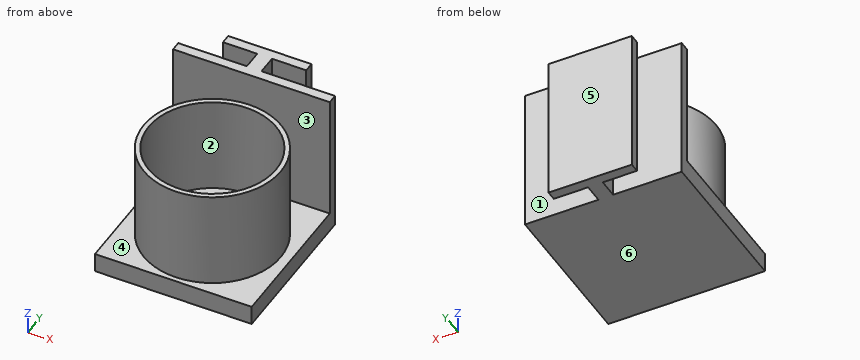
from build123d import *

# Parameters (mm, degrees)
F0_W     = 1.5
F0_H     = 2
F1_DEPTH = 15
F3_DEPTH = 1
F4_W     = 16
F4_H     = 2
F5_DEPTH = 15
F6_R     = 7
F6_R_2   = 6.5
F7_DEPTH = 10


with BuildPart() as f1:
    # F0 (on Top) → F1 (new body)
    with BuildSketch(Plane.XY):
        with Locations((4.5, 7)):
            Rectangle(F0_W, F0_H)
        Polygon((0.25, 8), (3.75, 8), (5.25, 8), (8.75, 8), (8.75, 9), (0.25, 9), align=None)
    extrude(amount=F1_DEPTH)

    # F2 (on face) → F3 (join)
    with BuildSketch(Plane.XZ.offset(-6)):
        Polygon((12.75, 15), (3.75, 15), (-3.25, 15), (-3.25, 0), (12.75, 0), align=None)
    extrude(amount=F3_DEPTH)

    # F4 (on face) → F5 (join)
    with BuildSketch(Plane.XZ.offset(-5)):
        with Locations((4.75, 1)):
            Rectangle(F4_W, F4_H)
    extrude(amount=F5_DEPTH)

    # F6 (on face) → F7 (join)
    with BuildSketch(Plane.XY.offset(2)):
        with Locations((4.75, -2.5)):
            Circle(F6_R)
        with Locations((4.75, -2.5)):
            Circle(F6_R_2, mode=Mode.SUBTRACT)
    extrude(amount=F7_DEPTH)


solid = f1.part
CAD build for the part. Positions are in the model's coordinates, mm. Face numbers are marked on the shaded views. A direction names the side the tool comes from. Round coordinates to 2 decimals unless told otherwise and drop trailing zeros. Write each loop counter-clockwise with the first axis right and the second up, starting at its lowest first coordinate (ties: lowest second). Pieces come first, ordered by that corner, then holes. Notation, with made-up numbers: M -29,54.5 L -9,54.5 A11 cw -9,60.5 Z; hole C 57.25,24 d9. An arc over 180 degrees is marked long. Use a Markdown table: item, result. Add a question column.
1. Slice it at C-C on y = -2.5. Give the cut face in (x, z).
2. Drill centre lines: probe 1 along Y at (x, z) = (4.75, 9.5); probe 2 along Y at (x, z) = (8.5, 14); probe 3 along Y at (x, z) = (2.25, 2.5). Where is each one in solid material? Low to high.
3. Slice it at A-A on z = 4.5. Give the cut face in (x, y), then the cut area to 3 significant figures.
4. Slice it at B-B on x = 8.25. Give the cut face in (y, z).
5. Flat gauge pins, fed straight in: P1, Ø7, axis at x = 1.5, y = -0.5, coming from the +Z side; P2, Ø1, axis at x = 2.5, z = 8.5, coming from the -Y side; P3, Ø4, axis at y = 1.5, z = 9.5, coming from the -X side. Where does each tip first touch, or does it go through?
6. 3-axis set-ups, long thin cutter, end or side, ignore diameter. For the marked faces 1, 2 and 3: which of +Z, -Z, +X, -X, +Y, -Y reach the whole face in a straight line?
7. Pull direction Y, two halves, no side cores. Call the marked faces 4, 5 and 6: released by +Y, released by -Y, zero draft, split by the parting line, or undercut.
8. Slice it at D-D on z = 13.25. Give the cut face in (x, y).
Reply:
| question | item | result |
|---|---|---|
| 1 | outline | M -3.25,0 L 12.75,0 L 12.75,2 L 11.75,2 L 11.75,12 L 11.25,12 L 11.25,2 L -1.75,2 L -1.75,12 L -2.25,12 L -2.25,2 L -3.25,2 Z |
| 2 | probe 1 | y = -9.5 to -9, 4 to 4.5, 5 to 9 |
| 2 | probe 2 | y = 5 to 6, 8 to 9 |
| 2 | probe 3 | y = -9.04 to -8.5, 3.5 to 4.04, 5 to 6, 8 to 9 |
| 3 | outline | M -3.25,5 L 12.75,5 L 12.75,6 L 5.25,6 L 5.25,8 L 8.75,8 L 8.75,9 L 0.25,9 L 0.25,8 L 3.75,8 L 3.75,6 L -3.25,6 Z; C 4.75,-2.5 d14; hole C 4.75,-2.5 d13 |
| 3 | area | 48.7 mm^2 |
| 4 | outline | M -10,0 L 6,0 L 6,15 L 5,15 L 5,2 L 3.56,2 L 3.56,12 L 2.98,12 L 2.98,2 L -7.98,2 L -7.98,12 L -8.56,12 L -8.56,2 L -10,2 Z; M 8,0 L 9,0 L 9,15 L 8,15 Z |
| 5 | P1 | stops at z = 12 |
| 5 | P2 | stops at y = -9.28 |
| 5 | P3 | stops at x = -1.96 |
| 6 | face 1 | +Z, -Z, +X |
| 6 | face 2 | +Z |
| 6 | face 3 | +Z, +X, -X |
| 7 | face 4 | undercut |
| 7 | face 5 | released by +Y |
| 7 | face 6 | zero draft |
| 8 | outline | M -3.25,5 L 12.75,5 L 12.75,6 L 5.25,6 L 5.25,8 L 8.75,8 L 8.75,9 L 0.25,9 L 0.25,8 L 3.75,8 L 3.75,6 L -3.25,6 Z |
